For this review, take the finished solid that the model builds, in its own axes (mm). A direction names the side the tool comes from. Give positions to 0.01 mm unless a question says otherwise; leave off trailing zeros. Loops run counter-clockwise (first coordinate to the right, second up) from the corner with the lowest first, then second, coordinate; pieces in that order, holes last. Notation, with made-up numbers: (85, 71.25) - (98, 71.25) arc R24 cw to (98, 109.25) - close; hole circle Ø8 at (-11.5, -39). An arc over 180 degrees is marked (long way). Use CSV: the item, a comma, the result in double quotes. Start each with the question number.
1. For faces 1 (the cylindrical face through (-4.454, -20.056, 87.325)), 2 (the cylindrical face through (-13.285, 12.182, 62.325)), list the 3-axis set-ups (+Z, -Z, +X, -X, +Y, -Y) from which the entire face can be reached by the end or side of a thin tool; tool diameter is ignored.
2. Wall thickness on line 1 (Z direction, x = -14.5, y = -12); line 2 (Z direction, x = 17, y = -15); line 3 (X direction, y = -17, z = 85): over which ranges is each line inside the solid? List them lowest first.
3. For pin 1 (5 mm diameter, centred on y = 1.5, z = 53, fed in from -X) (3 decimals); pin 2 (1 mm diameter, centred on y = 15, z = 80.5, fed in from -X); pin 3 (3 mm diameter, centred on y = 0, z = 102.5, fed in from +X), all flat-tipped, find the tip position at first contact; note any pin that passes through.
4. Take a section at A-A on x = 0. Give the boundary of the cut face in (y, z) (3 decimals).
5. Mouldability with a two-part tool opening along Z and no side actions: class faces 3 (the flat face through (0, 0, 0)), 4 (the flat face through (14, -12, 50)), 5 (the cylindrical face through (-14.31, -10.97, 112.32)) as pulls with the +Z half, pulls with the -Z half, needs draft (parallel to the pull), parting line crosses it, or undercut.
6. Take a section at C-C on z = 34. Give the boundary of the cut face in (x, y) (3 decimals).
```python
from build123d import *

# Parameters (mm, degrees)
F0_R     = 23.08
F1_DEPTH = 25
F2_R     = 23.115
F3_DEPTH = 25
F4_R     = 18.025
F5_DEPTH = 25
F6_R     = 20.545
F7_DEPTH = 25
F8_R     = 18.03
F9_DEPTH = 25


with BuildPart() as f1:
    # F0 (on Top) → F1 (new body)
    with BuildSketch(Plane.XY):
        Circle(F0_R)
    extrude(amount=F1_DEPTH)

    # F2 (on face) → F3 (join)
    with BuildSketch(Plane.XY.offset(25)):
        Circle(F2_R)
    extrude(amount=F3_DEPTH)

    # F4 (on face) → F5 (join)
    with BuildSketch(Plane.XY.offset(50)):
        Circle(F4_R)
    extrude(amount=F5_DEPTH)

    # F6 (on face) → F7 (join)
    with BuildSketch(Plane.XY.offset(75)):
        Circle(F6_R)
    extrude(amount=F7_DEPTH)

    # F8 (on face) → F9 (join)
    with BuildSketch(Plane.XY.offset(100)):
        Circle(F8_R)
    extrude(amount=F9_DEPTH)


solid = f1.part
```
Check result:
1,face 1,"+Z"
1,face 2,"none"
2,line 1,"z = 0 to 50, 75 to 100"
2,line 2,"z = 0 to 50"
2,line 3,"x = -11.54 to 11.54"
3,pin 1,"stops at x = -18.025"
3,pin 2,"stops at x = -14.55"
3,pin 3,"stops at x = 18.03"
4,outline,"(-23.115, 25) - (-23.08, 25) - (-23.08, 0) - (23.08, 0) - (23.08, 25) - (23.115, 25) - (23.115, 50) - (18.025, 50) - (18.025, 75) - (20.545, 75) - (20.545, 100) - (18.03, 100) - (18.03, 125) - (-18.03, 125) - (-18.03, 100) - (-20.545, 100) - (-20.545, 75) - (-18.025, 75) - (-18.025, 50) - (-23.115, 50) - close"
5,face 3,"pulls with the -Z half"
5,face 4,"undercut"
5,face 5,"needs draft"
6,outline,"circle Ø46.23 at (0, 0)"
